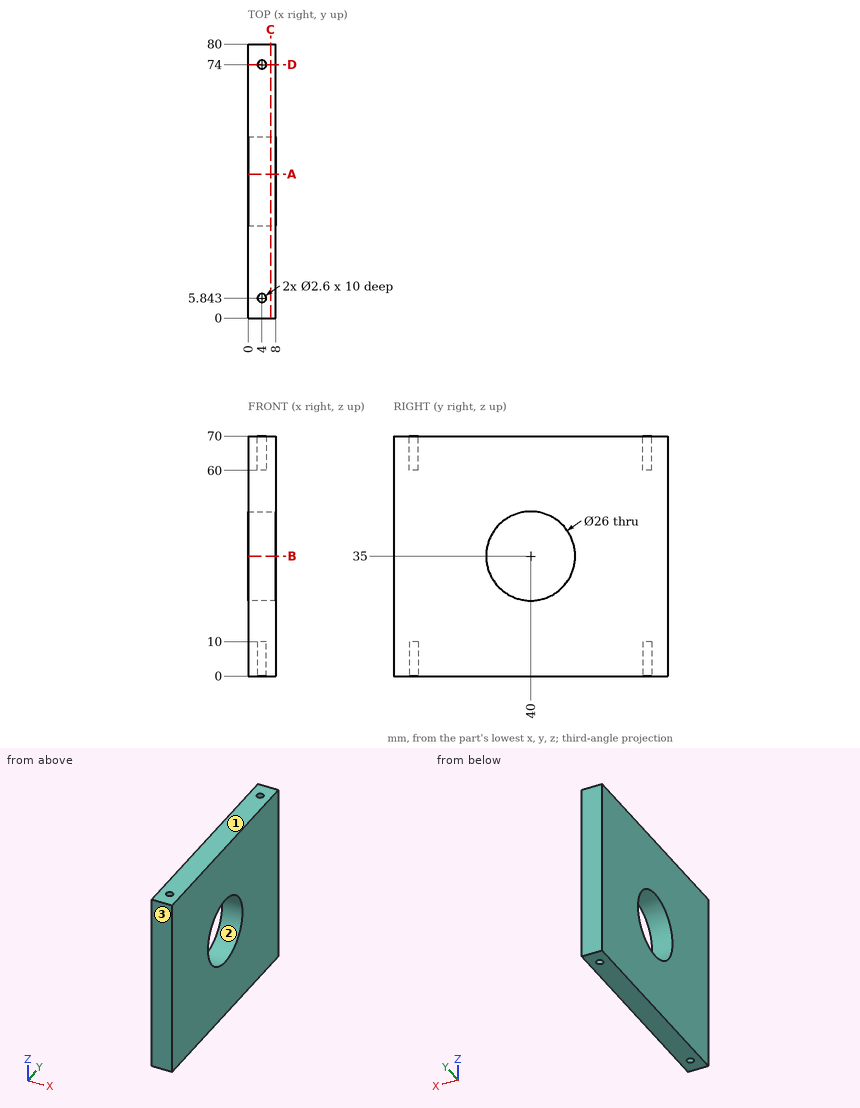
Answer from the drawing. Dimensions are ordinates in mm from the lowest x, y and z of the part. Give positions to 0.01 mm unless a question says otherwise; leave off trailing zeros. Loops run counter-clockwise (first coordinate to the right, second up) from the corner with the lowest first, then second, coordinate; pieces in that order, holes last.
Item 1: A cutting plane is placed at D-D (y = 74). Give the vertices of the cut face in (x, z), then the cut area to 3 significant figures.
Derived:
outline: (0, 0) - (2.7, 0) - (2.7, 10) - (5.3, 10) - (5.3, 0) - (8, 0) - (8, 70) - (5.3, 70) - (5.3, 60) - (2.7, 60) - (2.7, 70) - (0, 70) - close
area: 508 mm2
Item 2: Find the intervals of material crossed by line 1 along Y through (x, z) = (4, 7); line 2 along Y through (x, z) = (5.5, 39.5); line 3 along X through (y, z) = (74, 7), in increasing order.
Derived:
line 1: y = 0 to 4.54, 7.14 to 72.7, 75.3 to 80
line 2: y = 0 to 27.8, 52.2 to 80
line 3: x = 0 to 2.7, 5.3 to 8
Item 3: A cutting plane is placed at A-A (y = 42). Give the vertices of the cut face in (x, z) (1 decimal).
Derived:
outline: (0, 0) - (8, 0) - (8, 22.2) - (0, 22.2) - close; (0, 47.8) - (8, 47.8) - (8, 70) - (0, 70) - close
Item 4: A cutting plane is placed at C-C (x = 6.5). Give the vertices of the cut face in (y, z).
Derived:
outline: (0, 0) - (80, 0) - (80, 70) - (0, 70) - close; hole circle Ø26 at (40, 35)
Item 5: Determine the mould class of the marked faces 1, 2 and 3 for opening direction Y: +Y half, -Y half, draft (parallel to the pull), parting line (faces both ways), or undercut.
Derived:
face 1: draft
face 2: undercut
face 3: -Y half
Item 6: Each of these flat-tipped pins is pushed along its axis until it touches: pin 1 Ø2 at (x, y) = (4, 5.84) entering from +Z; pin 2 Ø1.3 at (x, y) = (4, 74.5) entering from -Z; pin 3 Ø15.5 at (y, z) = (40, 35) entering from -X. Where does it stop, or does it pass through?
Derived:
pin 1: stops at z = 60
pin 2: stops at z = 10
pin 3: passes through
Item 7: A cutting plane is placed at B-B (z = 35). Give the vertices of the cut face in (x, y), then the cut area to 3 significant figures.
Derived:
outline: (0, 0) - (8, 0) - (8, 27) - (0, 27) - close; (0, 53) - (8, 53) - (8, 80) - (0, 80) - close
area: 432 mm2
